```python
from build123d import *

# Parameters (mm, degrees)
F1_DEPTH = 6


with BuildPart() as f1:
    # F0 (on Front) → F1 (new body)
    with BuildSketch(Plane.XZ):
        with BuildLine():
            Line((0, 475), (0, 0))
            Line((0, 0), (2017, 0))
            Line((2017, 0), (2017, 475))
            Line((2017, 475), (1881.94281, 475))
            ThreePointArc((1881.94281, 475), (1861.14955, 440.987655), (1822, 448.505103))
            ThreePointArc((1822, 448.505103), (1782.85045, 440.987655), (1762.05719, 475))
            Line((1762.05719, 475), (329.94281, 475))
            ThreePointArc((329.94281, 475), (309.14955, 440.987655), (270, 448.505103))
            ThreePointArc((270, 448.505103), (230.85045, 440.987655), (210.05719, 475))
            Line((210.05719, 475), (0, 475))
        make_face()
        with BuildLine():
            ThreePointArc((62, 157), (97, 192), (132, 157))
            Line((132, 157), (132, 86))
            ThreePointArc((132, 86), (97, 51), (62, 86))
            Line((62, 86), (62, 157))
        make_face(mode=Mode.SUBTRACT)
    extrude(amount=F1_DEPTH)


solid = f1.part
```
Check sheet for the modelled part. Datum: model origin and axes. Units: mm. A direction names the side the tool comes from. Give positions to 0.01 mm unless a question says otherwise; leave off trailing zeros. Loops run counter-clockwise (first coordinate to the right, second up) from the corner with the lowest first, then second, coordinate; pieces in that order, holes last. Notation, with made-up numbers: M -32.75,-14.75 L -28.75,-14.75 A15 cw -28.75,3.25 Z; hole C 21,-40 d4. An arc over 180 degrees is marked long. Answer in a Markdown table with one row per item.
1) Cross-section at A-A (x = 97). Enter the section's corners in (y, z), plus the area to 3 significant figures.
Solutions:
| item | result |
|---|---|
| outline | M -6,0 L 0,0 L 0,51 L -6,51 Z; M -6,192 L 0,192 L 0,475 L -6,475 Z |
| area | 2,000 mm^2 |
2) Mould release check, pull along X, two halves, no side actions. Record for faces 3 (the face through (97.77, -2.96, 51.01)), 4 (the face through (994, -6, 241)): released by +X, released by -X, zero draft, split by the parting line, or undercut.
Solutions:
| item | result |
|---|---|
| face 3 | undercut |
| face 4 | zero draft |
3) Thickness scan on line 1 (X direction, y = -0.95, z = 139); line 2 (Z direction, x = 1803, y = -3.6). Record the ranges inside material, lowest first.
Solutions:
| item | result |
|---|---|
| line 1 | x = 0 to 62, 132 to 2017 |
| line 2 | z = 0 to 438.52 |
4) Cross-section at B-B (y = -4.75). Enter the section's corners in (x, z), plus the area to 3 significant figures.
Solutions:
| item | result |
|---|---|
| outline | M 0,0 L 2017,0 L 2017,475 L 1881.94,475 A35 cw 1822,448.51 A35 cw 1762.06,475 L 329.94,475 A35 cw 270,448.51 A35 cw 210.06,475 L 0,475 Z; hole M 62,86 A35 ccw 132,86 L 132,157 A35 ccw 62,157 Z |
| area | 942,000 mm^2 |
5) Tool access check on faces 1 (the face through (994, 0, 241)), 2 (the face through (96.23, -2.96, 191.99)). Record the directions out of +Z, -Z, +X, -X, +Y, -Y that give a thin tool (end or side, any length) a straight path to the whole face; none if there is none.
Solutions:
| item | result |
|---|---|
| face 1 | +Z, -Z, +X, -X, +Y |
| face 2 | +Y, -Y |
